Here's the drawing with two shaded views (mm, measured from the low corner). I have some questions. A direction names the side the tool comes from. Coordinates: 2 decimals unless noted, no trailing zeros. Loops run counter-clockwise (first coordinate to the right, second up) from the corner with the lowest first, then second, coordinate; pieces in that order, holes last.
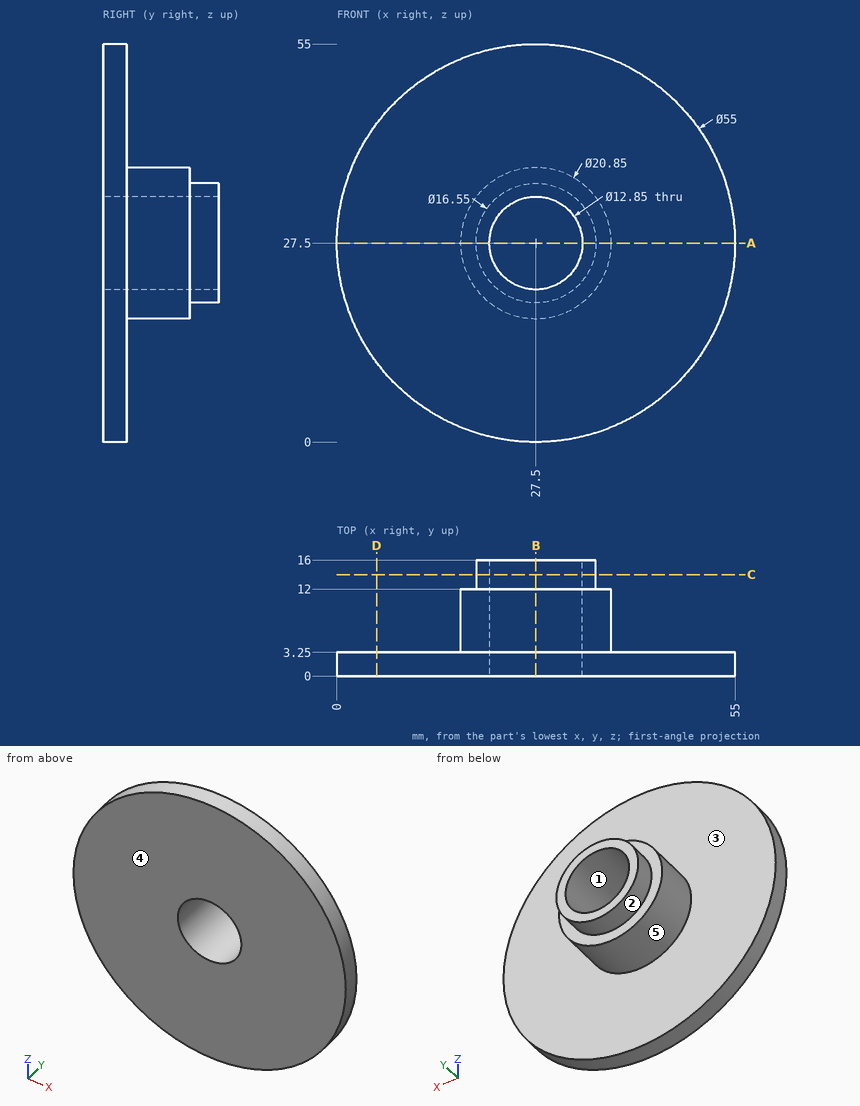
(1) If we mould it in two halves opening along X, with no side actions, what happens to the marked faces 1, 2 and 3? For each: released by +X, released by -X, zero draft, split by the parting line, or undercut.
Check values:
face 1: undercut
face 2: split by the parting line
face 3: zero draft
(2) I want a section at C-C on y = 14. Write out the boundary of the cut face in (x, z) (3 decimals), then the cut area to 3 significant figures.
Check values:
outline: circle Ø16.55 at (27.5, 27.5); hole circle Ø12.85 at (27.5, 27.5)
area: 85.4 mm2
(3) I want a section at B-B on x = 27.5. Write out the boundary of the cut face in (y, z) (3 decimals).
Check values:
outline: (0, 0) - (3.25, 0) - (3.25, 17.075) - (12, 17.075) - (12, 19.225) - (16, 19.225) - (16, 21.075) - (0, 21.075) - close; (0, 33.925) - (16, 33.925) - (16, 35.775) - (12, 35.775) - (12, 37.925) - (3.25, 37.925) - (3.25, 55) - (0, 55) - close
(4) I want a section at A-A on z = 27.5. Write out the boundary of the cut face in (x, y) (3 decimals), then the cut area to 3 significant figures.
Check values:
outline: (0, 0) - (21.075, 0) - (21.075, 16) - (19.225, 16) - (19.225, 12) - (17.075, 12) - (17.075, 3.25) - (0, 3.25) - close; (33.925, 0) - (55, 0) - (55, 3.25) - (37.925, 3.25) - (37.925, 12) - (35.775, 12) - (35.775, 16) - (33.925, 16) - close
area: 222 mm2
(5) If I drill on probe 1 along X at (y, z) = (4, 27.5) (3 decimals); probe 2 along Z at (x, y) = (27.5, 12.25) (3 decimals); probe 3 along Y at (x, z) = (39, 23), over which ranges is the centre line in solid material (lowest first)?
Check values:
probe 1: x = 17.075 to 21.075, 33.925 to 37.925
probe 2: z = 19.225 to 21.075, 33.925 to 35.775
probe 3: y = 0 to 3.25
(6) I want a section at D-D on x = 5.5. Write out the boundary of the cut face in (y, z).
Check values:
outline: (0, 11) - (3.25, 11) - (3.25, 44) - (0, 44) - close
(7) I'm going to push flat-ended pins straight in: pin 1 (1.5 mm diameter, centred on x = 46.5, z = 35.5, fed in from +Y); pin 2 (1.5 mm diameter, centred on x = 33, z = 36, fed in from +Y). Where does each tip first touch, or does it pass through?
Check values:
pin 1: stops at y = 3.25
pin 2: stops at y = 12
(8) Which directions (+Z, -Z, +X, -X, +Y, -Y) give clear straight access to the entire face, cutting with the end or side of a thin tool? Please do the marked faces 4 and 5.
Check values:
face 4: +Z, -Z, +X, -X, -Y
face 5: +Y
